Check sheet for the modelled part. Datum: model origin and axes. Units: mm. Face numbers are marked on the shaded views. Give positions to 0.01 mm unless a question says otherwise; leave off trailing zeros. Order: outer loops, then holes, each group sorted by start corner. A loop starts at its lowest first (then second) coordinate and runs counter-clockwise, first axis right, second up.
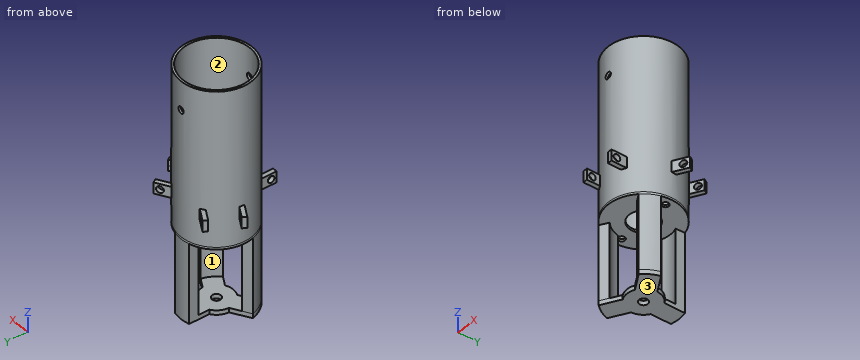
```python
from build123d import *

# Parameters (mm, degrees)
SKETCH1_R           = 16
SKETCH1_R_2         = 15
BOSS_EXTRUDE1_DEPTH = 70
BOSS_EXTRUDE2_START = 1
SKETCH3_R           = 16
BOSS_EXTRUDE2_DEPTH = 1
CUT_EXTRUDE2_REACH  = 76.518
SKETCH4_R           = 6.5
BOSS_EXTRUDE3_START = 34
BOSS_EXTRUDE3_DEPTH = 34
BOSS_EXTRUDE4_START = 2
SKETCH6_R           = 2
BOSS_EXTRUDE4_DEPTH = 2
BOSS_EXTRUDE5_DEPTH = 2.5
SKETCH8_R           = 1.5
CUT_EXTRUDE3_DEPTH  = 77.740858419
CIRPATTERN1_COUNT   = 3
SKETCH9_R           = 1.5
CUT_EXTRUDE4_DEPTH  = 78.206291301
SKETCH10_W          = 1.5
SKETCH10_H          = 40


with BuildPart() as part:
    # Sketch1 → Boss-Extrude1 (new body)
    with BuildSketch(Plane.XY):
        Circle(SKETCH1_R)
        Circle(SKETCH1_R_2, mode=Mode.SUBTRACT)
    extrude(amount=BOSS_EXTRUDE1_DEPTH)

    # Sketch3 → Boss-Extrude2 (add)
    with BuildSketch(Plane(origin=(0, 0, 0), x_dir=(-1, 0, 0), z_dir=(0, 0, -1)).offset(BOSS_EXTRUDE2_START)):
        Circle(SKETCH3_R)
    extrude(amount=-BOSS_EXTRUDE2_DEPTH)

    # Sketch4 → Cut-Extrude2 (cut, up to next)
    with BuildSketch(Plane(origin=(0, 0, -1), x_dir=(-1, 0, 0), z_dir=(0, 0, -1)), mode=Mode.PRIVATE) as cut_extrude2_sk1:
        Circle(SKETCH4_R)
    cut_extrude2_tool1 = extrude(cut_extrude2_sk1.sketch, amount=-CUT_EXTRUDE2_REACH, mode=Mode.PRIVATE) & part.part
    add(cut_extrude2_tool1.solids().sort_by_distance((0, 0, -1))[0], mode=Mode.SUBTRACT)

    # Sketch5 → Boss-Extrude3 (add)
    with BuildSketch(Plane(origin=(0, 0, -1), x_dir=(-1, 0, 0), z_dir=(0, 0, -1)).offset(BOSS_EXTRUDE3_START)):
        with BuildLine():
            Line((-4, 15.491933385), (-4, 11.313708499))
            ThreePointArc((-4, 11.313708499), (0, 12), (4, 11.313708499))
            Line((4, 11.313708499), (4, 15.491933385))
            ThreePointArc((4, 15.491933385), (0, 16), (-4, 15.491933385))
        make_face()
        with BuildLine():
            Line((15.416407865, -4.281865077), (11.797958971, -2.192752634))
            ThreePointArc((11.797958971, -2.192752634), (10.392304845, -6), (7.797958971, -9.120955865))
            Line((7.797958971, -9.120955865), (11.416407865, -11.210068308))
            ThreePointArc((11.416407865, -11.210068308), (13.856406461, -8), (15.416407865, -4.281865077))
        make_face()
        with BuildLine():
            Line((-11.416407865, -11.210068308), (-7.797958971, -9.120955865))
            ThreePointArc((-7.797958971, -9.120955865), (-10.392304845, -6), (-11.797958971, -2.192752634))
            Line((-11.797958971, -2.192752634), (-15.416407865, -4.281865077))
            ThreePointArc((-15.416407865, -4.281865077), (-13.856406461, -8), (-11.416407865, -11.210068308))
        make_face()
    extrude(amount=-BOSS_EXTRUDE3_DEPTH)

    # Sketch6 → Boss-Extrude4 (add)
    with BuildSketch(Plane(origin=(0, 0, -35), x_dir=(-1, 0, 0), z_dir=(0, 0, -1)).offset(BOSS_EXTRUDE4_START)):
        with BuildLine():
            Line((-4, 15.491933385), (-4, 6.34428877))
            ThreePointArc((-4, 6.34428877), (-6.495190528, 3.75), (-7.494315244, 0.29195723))
            Line((-7.494315244, 0.29195723), (-15.416407865, -4.281865077))
            ThreePointArc((-15.416407865, -4.281865077), (-13.856406461, -8), (-11.416407865, -11.210068308))
            Line((-11.416407865, -11.210068308), (-3.494315244, -6.636246))
            ThreePointArc((-3.494315244, -6.636246), (0, -7.5), (3.494315244, -6.636246))
            Line((3.494315244, -6.636246), (11.416407865, -11.210068308))
            ThreePointArc((11.416407865, -11.210068308), (13.856406461, -8), (15.416407865, -4.281865077))
            Line((15.416407865, -4.281865077), (7.494315244, 0.29195723))
            ThreePointArc((7.494315244, 0.29195723), (6.495190528, 3.75), (4, 6.34428877))
            Line((4, 6.34428877), (4, 15.491933385))
            ThreePointArc((4, 15.491933385), (0, 16), (-4, 15.491933385))
        make_face()
        Circle(SKETCH6_R, mode=Mode.SUBTRACT)
    extrude(amount=-BOSS_EXTRUDE4_DEPTH)

    # Sketch7 → Boss-Extrude5 (add, symmetric)
    with BuildSketch(Plane(origin=(0, 0, 14), x_dir=(-1, 0, 0), z_dir=(0, 0, -1))):
        with BuildLine():
            Line((15.041385001, 15.61235091), (9.845232579, 12.61235091))
            ThreePointArc((9.845232579, 12.61235091), (8.94427191, 13.266499161), (8, 13.856406461))
            Line((8, 13.856406461), (14.041385001, 17.344401717))
            Line((14.041385001, 17.344401717), (15.041385001, 15.61235091))
        make_face()
        with BuildLine():
            Line((21.041385001, 5.220046064), (22.041385001, 3.487995257))
            Line((22.041385001, 3.487995257), (16, 0))
            ThreePointArc((16, 0), (15.961261248, 1.112717112), (15.845232579, 2.220046064))
            Line((15.845232579, 2.220046064), (21.041385001, 5.220046064))
        make_face()
    boss_extrude5 = extrude(amount=BOSS_EXTRUDE5_DEPTH, both=True)

    # Sketch8 → Cut-Extrude3 (cut, through all)
    with BuildSketch(Plane(origin=(-4, -6.92820323, 0), x_dir=(0.8660254037844398, -0.49999999999999806, 0), z_dir=(-0.499999999999998, -0.8660254037844397, 0))):
        with Locations((-18.332396974, 14)):
            Circle(SKETCH8_R)
    cut_extrude3 = extrude(amount=-CUT_EXTRUDE3_DEPTH, mode=Mode.SUBTRACT)

    # CirPattern1: Boss-Extrude5, Cut-Extrude3 ×3 about axis
    cirpattern1_axis = Axis((0, 0, 0), (0, 0, 1))
    add([boss_extrude5.rotate(cirpattern1_axis, i * 360 / CIRPATTERN1_COUNT) for i in range(1, CIRPATTERN1_COUNT)])
    add([cut_extrude3.rotate(cirpattern1_axis, i * 360 / CIRPATTERN1_COUNT) for i in range(1, CIRPATTERN1_COUNT)], mode=Mode.SUBTRACT)

    # Sketch9 → Cut-Extrude4 (cut, through all)
    with BuildSketch(Plane(origin=(0, 0, -1), x_dir=(-1, 0, 0), z_dir=(0, 0, -1))):
        with Locations((-12.5, 0)):
            Circle(SKETCH9_R)
        with Locations((12.5, 0)):
            Circle(SKETCH9_R)
    extrude(amount=-CUT_EXTRUDE4_DEPTH, mode=Mode.SUBTRACT)

    # Sketch10 → Cut-Revolve1 (revolve, cut)
    with BuildSketch(Plane.XY.offset(57), mode=Mode.PRIVATE) as cut_revolve1_sk:
        with Locations((0.75, 0)):
            Rectangle(SKETCH10_W, SKETCH10_H)
    revolve(cut_revolve1_sk.sketch.rotate(Axis((0, 0, 57), (0, 1, 0)), 90), axis=Axis((0, 0, 57), (0, 1, 0)), mode=Mode.SUBTRACT)


solid = part.part
```
Q1. Material ranges on line 1 (Z direction, x = 10.5, y = -4); line 2 (Y direction, x = 0, z = 32.5); line 3 (Y direction, x = 0, z = -0.6), recorded low to high.
Q2. Go/stop test with flat-tipped pins: P1, Ø1.8, axis at x = 12.5, y = 0, coming from the +Z side; P2, Ø15, axis at x = -1.5, y = -2.5, coming from the +Z side; P3, Ø5.5, axis at y = -19, z = 14.5, coming from the +X side; P4, Ø2.5, axis at x = 18, y = 2.5, coming from the -Z side. Record where each tip stops, or that it passes through.
Q3. Sectioned sample at B-B, the plane y = 10. Record the cut outline in (x, z), plus the area to 3 significant figures.
Q4. Draft check along Y on the marked faces 1, 2 and 3. Enter one of: pulls with the +Y half, pulls with the -Y half, needs draft (parallel to the pull), parting line crosses it, or undercut.
Q5. Sectioned sample at C-C, the plane x = -13. Count the separate pieces of the cut face and the enclosed holes in it, plus the area to 3 significant figures.
Filled in:
1. line 1: z = -37 to -35, -1 to 0
1. line 2: y = -16 to -15, 15 to 16
1. line 3: y = -16 to -6.5, 6.5 to 16
2. P1: passes through
2. P2: stops at z = 0
2. P3: stops at x = 8
2. P4: stops at z = 11.5
3. outline: (-12.49, -1) - (12.49, -1) - (12.49, 70) - (11.18, 70) - (11.18, 0) - (-11.18, 0) - (-11.18, 70) - (-12.49, 70) - close; (-4, -37) - (4, -37) - (4, -35) - (-4, -35) - close
3. area: 224 mm2
4. face 1: pulls with the +Y half
4. face 2: undercut
4. face 3: needs draft
5. separate pieces: 4
5. enclosed holes: 0
5. area: 512 mm2
